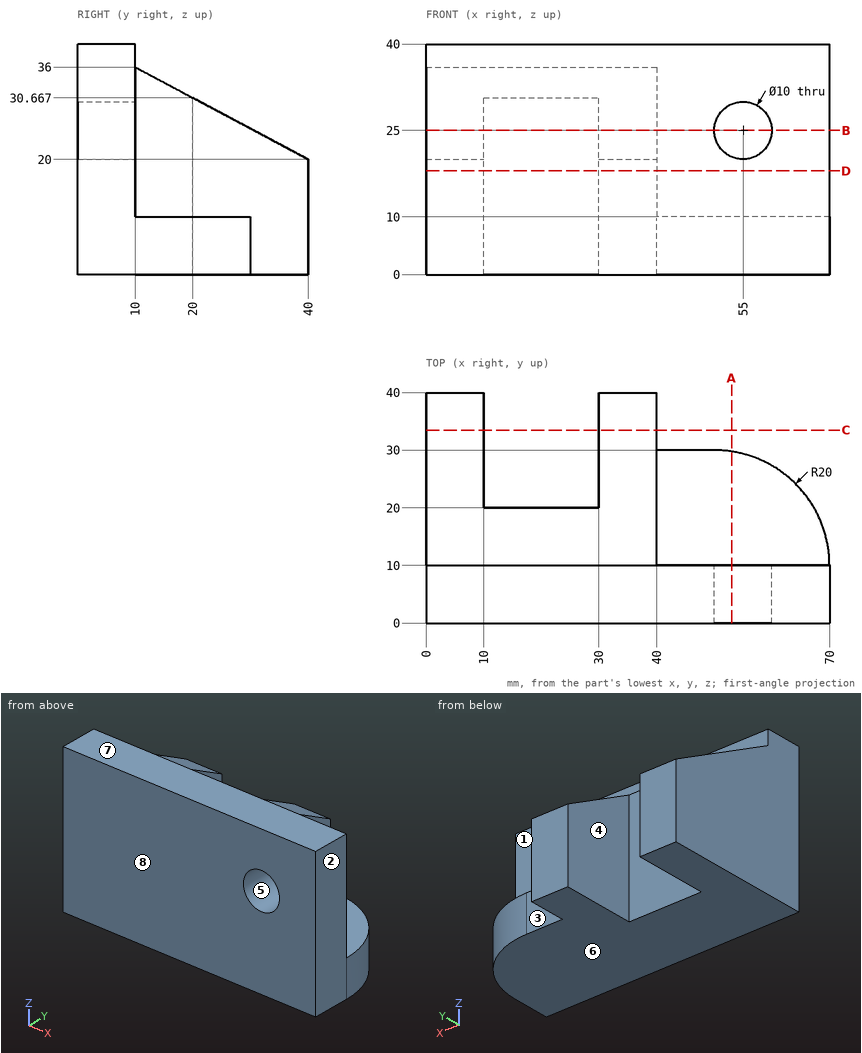
Geometry: see drawing. Coordinates: mm, zero at the bounding-box minimum. A direction names the side the tool comes from. Coordinates: 2 decimals unless noted, no trailing zeros. Loops run counter-clockwise (first coordinate to the right, second up) from the corner with the lowest first, then second, coordinate; pieces in that order, holes last.
Q1. Contact query for flat-ended pins moving along their axis: pin 1 (2 mm diameter, centred on x = 49.5, z = 34, fed in from +Y); pin 2 (3 mm diameter, centred on y = 16, z = 29, fed in from +X); pin 3 (5 mm diameter, centred on x = 8, y = 25.5, fed in from +Z). Output: stop coordinate, or through.
Q2. Material intervals for line 1 (Z direction, x = 55, y = 2); line 2 (X direction, y = 24, z = 19); line 3 (X direction, y = 7.25, z = 25), sorted ascending.
Q3. Cut plane A-A (x = 53). Output: boundary loops of the cut face in (y, z), then the cut area to 3 significant figures.
Q4. Cut plane D-D (z = 18). Output: boundary loops of the cut face in (x, y).
Q5. Draft query along Z for the marked faces 5, 6, 7 and 8. Return one class per face: +Z half, -Z half, draft (parallel to the pull), parting line (faces both ways), or undercut.
Q6. Cut plane C-C (y = 33.5). Output: boundary loops of the cut face in (x, z), then the cut area to 3 significant figures.
Q7. Set-up query: the marked faces 1, 2, 3 and 4. Return all of +Z, -Z, +X, -X, +Y, -Y with unobstructed straight access to the full face (end or side cutting, diameter ignored); none if empty.
Q8. Cut plane B-B (z = 25). Output: boundary loops of the cut face in (x, y) (1 decimal), then the cut area to 3 significant figures.
Working result:
1. pin 1: stops at y = 10
1. pin 2: stops at x = 40
1. pin 3: stops at z = 29.07
2. line 1: z = 0 to 20, 30 to 40
2. line 2: x = 0 to 10, 30 to 40
2. line 3: x = 0 to 50, 60 to 70
3. outline: (0, 0) - (29.77, 0) - (29.77, 10) - (10, 10) - (10, 20.42) - (0, 20.42) - close; (0, 29.58) - (10, 29.58) - (10, 40) - (0, 40) - close
3. area: 506 mm2
4. outline: (0, 0) - (70, 0) - (70, 10) - (40, 10) - (40, 40) - (30, 40) - (30, 20) - (10, 20) - (10, 40) - (0, 40) - close
5. face 5: undercut
5. face 6: -Z half
5. face 7: +Z half
5. face 8: draft
6. outline: (0, 0) - (10, 0) - (10, 23.47) - (0, 23.47) - close; (30, 0) - (40, 0) - (40, 23.47) - (30, 23.47) - close
6. area: 469 mm2
7. face 1: +Z, +X, +Y
7. face 2: +Z, -Z, +X, +Y, -Y
7. face 3: +Z, -Z, +X, +Y
7. face 4: +Z, -Z, +Y
8. outline: (0, 0) - (50, 0) - (50, 10) - (40, 10) - (40, 30.6) - (30, 30.6) - (30, 20) - (10, 20) - (10, 30.6) - (0, 30.6) - close; (60, 0) - (70, 0) - (70, 10) - (60, 10) - close
8. area: 1,210 mm2
